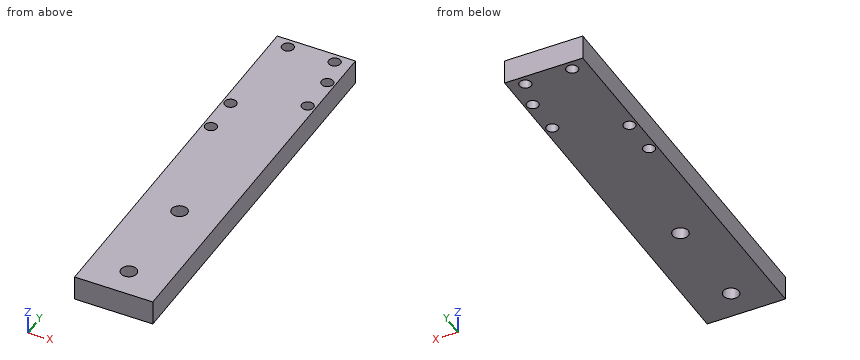
from build123d import *

# Parameters (mm, degrees)
SKETCH1_W           = 20
SKETCH1_H           = 40
SKETCH1_R           = 2
BOSS_EXTRUDE1_DEPTH = 6.35
SKETCH3_W           = 20
SKETCH3_H           = 6.35
BOSS_EXTRUDE3_DEPTH = 60
SKETCH6_R           = 1.5
CUT_EXTRUDE1_DEPTH  = 23.2


with BuildPart() as part:
    # Sketch1 → Boss-Extrude1 (new body)
    with BuildSketch(Plane.XY):
        with Locations((10, 20)):
            Rectangle(SKETCH1_W, SKETCH1_H)
        with Locations((10, 32.5)):
            Circle(SKETCH1_R, mode=Mode.SUBTRACT)
        with Locations((10, 7.5)):
            Circle(SKETCH1_R, mode=Mode.SUBTRACT)
    extrude(amount=BOSS_EXTRUDE1_DEPTH)

    # Sketch3 → Boss-Extrude3 (add)
    with BuildSketch(Plane(origin=(0, 40, 0), x_dir=(1, 0, 0), z_dir=(0, 1, 0))):
        with Locations((10, -3.175)):
            Rectangle(SKETCH3_W, SKETCH3_H)
    extrude(amount=BOSS_EXTRUDE3_DEPTH)

    # Sketch6 → Cut-Extrude1 (cut)
    with BuildSketch(Plane(origin=(0, 0, 0), x_dir=(-1, 0, 0), z_dir=(0, 0, -1))):
        with Locations((-16, 97.5)):
            Circle(SKETCH6_R)
        with Locations((-4, 97.5)):
            Circle(SKETCH6_R)
        with Locations((-18, 90)):
            Circle(SKETCH6_R)
        with Locations((-2, 63.448163905)):
            Circle(SKETCH6_R)
        with Locations((-2, 73.131019592)):
            Circle(SKETCH6_R)
        with Locations((-18, 80.317144313)):
            Circle(SKETCH6_R)
    extrude(amount=-CUT_EXTRUDE1_DEPTH, mode=Mode.SUBTRACT)


solid = part.part
The model under review builds one solid part; all positions refer to its coordinate system, in mm. Round coordinates to 2 decimals unless told otherwise and drop trailing zeros. Order: outer loops, then holes, each group sorted by start corner. A loop starts at its lowest first (then second) coordinate and runs counter-clockwise, first axis right, second up. Notation, with made-up numbers: (-35, 75.5) -> (3, 75.5) arc R19 cw to (3, 107.5) -> close; hole circle Ø10 at (-37, 48). An arc over 180 degrees is marked (long way). Use CSV: the item, a comma, the result in double quotes. Start each with the question number.
(1) Consider section B-B on x = 10. Write out the cut boundary in (y, z), and give its area (3 significant figures).
(2) Wall thickness on probe 1 along Y at (x, z) = (10, 1.5); probe 2 along Y at (x, z) = (18, 4.75); probe 3 along X at (y, z) = (97.5, 4.75): over which ranges is each line inside the solid? List them lowest first. Write a range as from..to.
(3) Consider section C-C on z = 4.5. State how many separate pieces and enclosed holes the cut face has, and give its area (3 significant figures).
(4) Consider section A-A on y = 97.5. Write out the cut boundary in (x, z).
Responses:
1,outline,"(0, 0) -> (5.5, 0) -> (5.5, 6.35) -> (0, 6.35) -> close; (9.5, 0) -> (30.5, 0) -> (30.5, 6.35) -> (9.5, 6.35) -> close; (34.5, 0) -> (100, 0) -> (100, 6.35) -> (34.5, 6.35) -> close"
1,area,"584 mm²"
2,probe 1,"0..5.5, 9.5..30.5, 34.5..100"
2,probe 2,"0..78.82, 81.82..88.5, 91.5..100"
2,probe 3,"0..2.5, 5.5..14.5, 17.5..20"
3,separate pieces,"1"
3,enclosed holes,"8"
3,area,"1,930 mm²"
4,outline,"(0, 0) -> (2.5, 0) -> (2.5, 6.35) -> (0, 6.35) -> close; (5.5, 0) -> (14.5, 0) -> (14.5, 6.35) -> (5.5, 6.35) -> close; (17.5, 0) -> (20, 0) -> (20, 6.35) -> (17.5, 6.35) -> close"
